from build123d import *

# Parameters (mm, degrees)
SKETCH009_R     = 4
PAD002_DEPTH    = 40
PAD004_DEPTH    = 21
POCKET007_DEPTH = 24


with BuildPart() as part:
    # Sketch009 → Pad002 (new body)
    with BuildSketch(Plane.YZ):
        Circle(SKETCH009_R)
    extrude(amount=PAD002_DEPTH)

    # Sketch011 → Pad004 (join)
    with BuildSketch(Plane.YZ):
        with BuildLine():
            ThreePointArc((1.9, 1.296148), (-2.3, 0), (1.9, -1.296148))
            Line((1.9, -0.65), (1.9, -1.296148))
            Line((1.4, -0.65), (1.9, -0.65))
            Line((1.4, 0.65), (1.4, -0.65))
            Line((1.9, 0.65), (1.4, 0.65))
            Line((1.9, 1.296148), (1.9, 0.65))
        make_face()
    extrude(amount=-PAD004_DEPTH)

    # Sketch021 (on Face3 of Pad004) → Pocket007 (cut)
    with BuildSketch(Plane.YZ.offset(40)):
        with BuildLine():
            Line((1.4, -1), (1.4, 1))
            Line((1.4, 1), (2.7, 1))
            Line((2.7, 1), (2.7, 2.951271))
            ThreePointArc((2.7, -2.951271), (4, 0), (2.7, 2.951271))
            Line((2.7, -1), (2.7, -2.951271))
            Line((1.4, -1), (2.7, -1))
        make_face()
    extrude(amount=-POCKET007_DEPTH, mode=Mode.SUBTRACT)


with BuildPart() as part_1:
    # Body002 placement: moved
    add(part.part.moved(Location((22, 0, 0))))


solid = part_1.part
Design review of the part built by this model. Coordinates are the model's own, in mm. A direction names the side the tool comes from. Round coordinates to 2 decimals unless told otherwise and drop trailing zeros. Loops run counter-clockwise (first coordinate to the right, second up) from the corner with the lowest first, then second, coordinate; pieces in that order, holes last. Notation, with made-up numbers: (68.5, 33) - (114.5, 33) arc R34 cw to (114.5, 68) - close; hole circle Ø5 at (76, 40.5). An arc over 180 degrees is marked (long way). One line per item, written item: value. Start each with the question number.
1) Insertion check: pin 1 Ø1 at (x, y) = (10, 0) entering from +Z; pin 2 Ø2 at (x, y) = (52, 1.5) entering from +Z; pin 3 Ø4 at (x, y) = (19.5, 0.5) entering from -Z. Each pin has a flat end and moves straight along its axis. Give the tip position at first contact, or say it passes through.
2) Consider section D-D on x = 17. Give the boundary of the cut face in (y, z), then the cut area to 3 significant figures.
3) Consider section A-A on y = 0. Give the boundary of the cut face in (x, z), then the cut area to 3 significant figures.
4) To check wall thickness, follow L1, parallel to X at y = 2, z = 1.25; L2, parallel to Y at x = 54, z = 0; L3, parallel to Z at x = 48.5, y = -0.5. State the ranges of each line that lie inside material, in increasing order. Write a range as from..to.
5) For faces 4 (the flat face through (1, 0, 0)), 5 (the flat face through (50, 2.7, -2)), 6 (the flat face through (50, 1.4, 0)), 7 (the cylindrical face through (42, -4, 0)), 8 (the flat face through (12, 1.4, 0)), list the 3-axis set-ups (+Z, -Z, +X, -X, +Y, -Y) from which the entire face can be reached by the end or side of a thin tool; tool diameter is ignored.
6) Consider section B-B on z = 0. Give the boundary of the cut face in (x, y).
7) Draft analysis for pull direction Z (two halves, no side actions). For faces 1 (the flat face through (50, 2.7, 2)), 2 (the cylindrical face through (11.65, -2.3, 0.08)), 3 (the flat face through (50, 2, 1)), state which applies: +Z half, -Z half, draft (parallel to the pull), parting line (faces both ways), or undercut.
8) Consider section C-C on x = 55.5. Give the boundary of the cut face in (y, z).
Reported:
1. pin 1: stops at z = 2.3
1. pin 2: stops at z = 3.97
1. pin 3: stops at z = -2.3
2. outline: (1.4, -0.65) - (1.4, 0.65) - (1.9, 0.65) - (1.9, 1.3) arc R2.3 ccw (long way) to (1.9, -1.3) - (1.9, -0.65) - close
2. area: 15.3 mm^2
3. outline: (1, -2.3) - (22, -2.3) - (22, -4) - (62, -4) - (62, 4) - (22, 4) - (22, 2.3) - (1, 2.3) - close
3. area: 417 mm^2
4. L1: x = 22..62
4. L2: y = -4..1.4
4. L3: z = -3.97..3.97
5. face 4: +Z, -Z, -X, +Y, -Y
5. face 5: +Z, -Z, +X, +Y
5. face 6: +X, +Y
5. face 7: +X, -X
5. face 8: -X, +Y
6. outline: (1, -2.3) - (22, -2.3) - (22, -4) - (62, -4) - (62, 1.4) - (38, 1.4) - (38, 4) - (22, 4) - (22, 1.4) - (1, 1.4) - close
7. face 1: draft
7. face 2: parting line
7. face 3: undercut
8. outline: (1.4, -1) - (1.4, 1) - (2.7, 1) - (2.7, 2.95) arc R4 ccw (long way) to (2.7, -2.95) - (2.7, -1) - close
